Check sheet for the modelled part. Datum: model origin and axes. Units: mm. Face numbers are marked on the shaded views. A direction names the side the tool comes from. Round coordinates to 2 decimals unless told otherwise and drop trailing zeros. Order: outer loops, then holes, each group sorted by start corner. A loop starts at its lowest first (then second) coordinate and runs counter-clockwise, first axis right, second up.
(1) Sectioned sample at B-B, the plane x = 22. Enter the section's corners in (y, z), and give its area (3 significant figures).
(2) Sectioned sample at A-A, the plane y = 74.5. Enter the section's corners in (x, z), and give its area (3 significant figures).
(3) Thickness scan on probe 1 along Z at (x, y) = (22, 72.4); probe 2 along Z at (x, y) = (22, 78.2); probe 3 along Y at (x, z) = (28, -6). Record the ranges inside material, lowest first.
(4) Depth check by flat-ended pin: pin 1 (12 mm diameter, centred on x = 30.5, z = -29, fed in from -Y); pin 2 (2 mm diameter, centred on x = 24, y = 62, fed in from -Z); pin 3 (2.5 mm diameter, centred on x = 24, z = -33, fed in from -Y); pin 4 (3.5 mm diameter, centred on x = 22, z = -33, fed in from -Y). Enter the tip coordinate at first touch or a pass-through.
(5) Sectioned sample at C-C, the plane z = -33. Enter the section's corners in (x, y), and give its area (3 significant figures).
(6) Tool access check on the marked faces 5 and 6. Record the directions out of +Z, -Z, +X, -X, +Y, -Y that give a thin tool (end or side, any length) a straight path to the whole face; none if there is none.
(7) Mould release check, pull along X, two halves, no side actions. Record for the marked faces 1, 2, 3 and 4: released by +X, released by -X, zero draft, split by the parting line, or undercut.
(8) Sectioned sample at D-D, the plane x = 32.5. Enter the section's corners in (y, z).
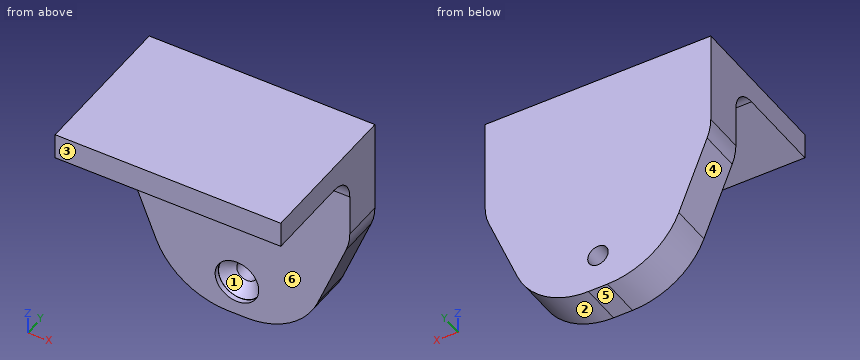
```python
from build123d import *

# Parameters (mm, degrees)
CYLINDER004_R             = 2
CYLINDER004_DEPTH         = 10
CYLINDER005_R             = 4.25
CYLINDER005_DEPTH         = 10
FUSION006_PLACEMENT_ANGLE = 180
CYLINDER006_R             = 4.25
CYLINDER006_DEPTH         = 10
CYLINDER003_R             = 2
CYLINDER003_DEPTH         = 10
CYLINDER002_R             = 4.25
CYLINDER002_DEPTH         = 10
EXTRUDE_DEPTH             = 8
BOX004_W                  = 24
BOX004_H                  = 8
BOX004_DEPTH              = 45
BOX003_W                  = 44
BOX003_H                  = 8
BOX003_DEPTH              = 15
BOX002_W                  = 44
BOX002_H                  = 30
BOX002_DEPTH              = 5
FILLET_R                  = 5
FILLET001_R               = 15
FILLET002_R               = 10
CHAMFER001_SIZE           = 2.2
CHAMFER002_SIZE           = 2.2


with BuildPart() as cylinder004:
    # Cylinder004 → Cylinder004 (new body)
    with BuildSketch(Plane(origin=(22, 80, -33), x_dir=(1, 0, 0), z_dir=(0, -1, 0))):
        Circle(CYLINDER004_R)
    extrude(amount=CYLINDER004_DEPTH)


with BuildPart() as fusion006:
    # Cylinder005 → Cylinder005 (new body)
    with BuildSketch(Plane(origin=(22, 89, -33), x_dir=(1, 0, 0), z_dir=(0, -1, 0))):
        Circle(CYLINDER005_R)
    extrude(amount=CYLINDER005_DEPTH)

    # Fusion006: union Cylinder004
    add(cylinder004.part)


with BuildPart() as fusion006_1:
    # Fusion006 placement: moved
    add(fusion006.part.moved(Location((0, 152, -66))).rotate(Axis((0, 152, -66), (1, 0, 0)), FUSION006_PLACEMENT_ANGLE))


with BuildPart() as cylinder006:
    # Cylinder006 → Cylinder006 (new body)
    with BuildSketch(Plane(origin=(22, 80, -33), x_dir=(1, 0, 0), z_dir=(0, -1, 0))):
        Circle(CYLINDER006_R)
    extrude(amount=CYLINDER006_DEPTH)


with BuildPart() as cylinder003:
    # Cylinder003 → Cylinder003 (new body)
    with BuildSketch(Plane(origin=(22, 80, -33), x_dir=(1, 0, 0), z_dir=(0, -1, 0))):
        Circle(CYLINDER003_R)
    extrude(amount=CYLINDER003_DEPTH)


with BuildPart() as fusion005:
    # Cylinder002 → Cylinder002 (new body)
    with BuildSketch(Plane(origin=(22, 89, -33), x_dir=(1, 0, 0), z_dir=(0, -1, 0))):
        Circle(CYLINDER002_R)
    extrude(amount=CYLINDER002_DEPTH)

    # Fusion005: union Cylinder003
    add(cylinder003.part)


with BuildPart() as extrude_body:
    # Sketch (on Face11 of Fusion003) → Extrude (new body)
    with BuildSketch(Plane(origin=(0, 80, 0), x_dir=(-1, 0, 0), z_dir=(0, 1, 0))):
        Polygon((-44, -15), (-34, -40), (-34, -15), align=None)
        Polygon((-10, -15), (0, -15), (-10, -40), align=None)
    extrude(amount=-EXTRUDE_DEPTH)


with BuildPart() as cube004:
    # Box004 → Box004 (new body)
    with BuildSketch(Plane(origin=(10, 72, -40), x_dir=(1, 0, 0), z_dir=(0, 0, 1))):
        with Locations((12, 4)):
            Rectangle(BOX004_W, BOX004_H)
    extrude(amount=BOX004_DEPTH)


with BuildPart() as cube003:
    # Box003 → Box003 (new body)
    with BuildSketch(Plane(origin=(0, 72, -15), x_dir=(1, 0, 0), z_dir=(0, 0, 1))):
        with Locations((22, 4)):
            Rectangle(BOX003_W, BOX003_H)
    extrude(amount=BOX003_DEPTH)


with BuildPart() as pieza_interior_x4:
    # Box002 → Box002 (new body)
    with BuildSketch(Plane(origin=(0, 50, 0), x_dir=(1, 0, 0), z_dir=(0, 0, 1))):
        with Locations((22, 15)):
            Rectangle(BOX002_W, BOX002_H)
    extrude(amount=BOX002_DEPTH)

    # Fusion002: union Cube003
    add(cube003.part)

    # Fillet
    fillet_edges = [pieza_interior_x4.edges().sort_by_distance(p)[0] for p in [
        (22, 72, 0),
    ]]
    fillet(fillet_edges, radius=FILLET_R)

    # Fusion003: union Cube004
    add(cube004.part)

    # Fusion004: union Extrude body
    add(extrude_body.part)

    # Fillet001
    fillet001_edges = [pieza_interior_x4.edges().sort_by_distance(p)[0] for p in [
        (10, 76, -40),
        (34, 76, -40),
    ]]
    fillet(fillet001_edges, radius=FILLET001_R)

    # Fillet002
    fillet002_edges = [pieza_interior_x4.edges().sort_by_distance(p)[0] for p in [
        (44, 76, -15),
        (0, 76, -15),
    ]]
    fillet(fillet002_edges, radius=FILLET002_R)

    # Cut001: cut Fusion005
    add(fusion005.part, mode=Mode.SUBTRACT)

    # Chamfer001
    chamfer001_edges = [pieza_interior_x4.edges().sort_by_distance(p)[0] for p in [
        (20, 79, -33),
    ]]
    chamfer(chamfer001_edges, length=CHAMFER001_SIZE)

    # Fusion007: union Cylinder006
    add(cylinder006.part)

    # Cut002: cut Fusion006
    add(fusion006_1.part, mode=Mode.SUBTRACT)

    # Chamfer002
    chamfer002_edges = [pieza_interior_x4.edges().sort_by_distance(p)[0] for p in [
        (20, 73, -33),
    ]]
    chamfer(chamfer002_edges, length=CHAMFER002_SIZE)


solid = pieza_interior_x4.part
```
Derived:
1. outline: (50, 0) - (67, 0) arc R5 cw to (72, -5) - (72, -28.75) - (73, -28.75) - (73, -28.8) - (75.2, -31) - (80, -31) - (80, 5) - (50, 5) - close; (72, -40) - (80, -40) - (80, -35) - (75.2, -35) - (73, -37.2) - (73, -37.25) - (72, -37.25) - close
1. area: 434 mm2
2. outline: (0, -13.07) arc R10 ccw to (0.72, -16.79) - (6.23, -30.57) arc R15 ccw to (20.16, -40) - (23.84, -40) arc R15 ccw to (37.77, -30.57) - (43.28, -16.79) arc R10 ccw to (44, -13.07) - (44, 5) - (0, 5) - close; hole circle Ø5.4 at (22, -33)
2. area: 1,670 mm2
3. probe 1: z = -40 to -37.25, -28.75 to 5
3. probe 2: z = -40 to -35, -31 to 5
3. probe 3: y = 72 to 80
4. pin 1: stops at y = 72
4. pin 2: stops at z = 0
4. pin 3: stops at y = 73.95
4. pin 4: passes through
5. outline: (7.47, 72) - (17.75, 72) - (17.75, 73) - (17.8, 73) - (20, 75.2) - (20, 80) - (7.47, 80) - close; (24, 75.2) - (26.2, 73) - (26.25, 73) - (26.25, 72) - (36.53, 72) - (36.53, 80) - (24, 80) - close
5. area: 191 mm2
6. face 5: -Z, +X, -X, +Y, -Y
6. face 6: -Z, +X, -X, -Y
7. face 1: undercut
7. face 2: released by +X
7. face 3: zero draft
7. face 4: released by -X
8. outline: (50, 0) - (67, 0) arc R5 cw to (72, -5) - (72, -37.25) - (80, -37.25) - (80, 5) - (50, 5) - close
